```python
from build123d import *

# Parameters (mm, degrees)
SKETCH_1_W          = 1780
SKETCH_1_H          = 100
SKETCH_1_R          = 13
EXTRUDE_573_DEPTH   = 8
SKETCH_2_W          = 1780
SKETCH_2_H          = 8
EXTRUDE_1_DEPTH     = 100
CUT_EXTRUDE_1_DEPTH = 903.088687436


with BuildPart() as part:
    # 草图1 → Extrude 573 (new body)
    with BuildSketch(Plane.XY):
        with Locations((0, 50)):
            Rectangle(SKETCH_1_W, SKETCH_1_H)
        with Locations((840, 40)):
            Circle(SKETCH_1_R, mode=Mode.SUBTRACT)
        with Locations((760, 40)):
            Circle(SKETCH_1_R, mode=Mode.SUBTRACT)
        with Locations(Location((-840, 40, 0), (0, 0, 180))):
            Circle(SKETCH_1_R, mode=Mode.SUBTRACT)
        with Locations(Location((-760, 40, 0), (0, 0, 180))):
            Circle(SKETCH_1_R, mode=Mode.SUBTRACT)
    extrude(amount=EXTRUDE_573_DEPTH)

    # 草图2 → 凸台-拉伸1 (add)
    with BuildSketch(Plane.XY.offset(8)):
        with Locations((0, 96)):
            Rectangle(SKETCH_2_W, SKETCH_2_H)
    extrude(amount=EXTRUDE_1_DEPTH)

    # 草图3 → 切除-拉伸1 (cut, through all)
    with BuildSketch(Plane(origin=(0, 100, 0), x_dir=(-1, 0, 0), z_dir=(0, 1, 0))):
        Polygon((-650, 108), (-890, 0), (-890, 108), align=None)
        Polygon((890, 108), (650, 108), (890, 0), align=None)
    extrude(amount=-CUT_EXTRUDE_1_DEPTH, mode=Mode.SUBTRACT)


solid = part.part
```
Here's how the part is built. I have some questions about the finished solid (model axes, mm). A direction names the side the tool comes from. Coordinates: 2 decimals unless noted, no trailing zeros. Write each loop counter-clockwise with the first axis right and the second up, starting at its lowest first coordinate (ties: lowest second). Pieces come first, ordered by that corner, then holes. Notation, with made-up numbers: (18, -2) - (63, -2) arc R18 cw to (63, 2) - close; hole circle Ø11 at (8, 36). An arc over 180 degrees is marked (long way). One line per item, written item: value.
1) I'm going to push flat-ended pins straight in: P1, Ø3, axis at x = -18.5, z = 67, coming from the -Y side; P2, Ø6, axis at x = 11, y = 59.5, coming from the +Z side. Where does each tip first touch, or does it pass through?
Model answer:
P1: stops at y = 92
P2: stops at z = 8
2) Suppose I cut it at C-C on z = 92. Write out the boundary of the cut face in (x, y), and give its area (3 significant figures).
Model answer:
outline: (-685.56, 92) - (685.56, 92) - (685.56, 100) - (-685.56, 100) - close
area: 11,000 mm²
3) On a 3-axis mill with a long thin cutter (end or side, diameter ignored), from which of +Z, -Z, +X, -X, +Y, -Y can I reach the whole of each face in a straight line? I mean faces 1 (the flat face through (-822.773, 94.678, 30.252)), 2 (the flat face through (-12, 92, 57)). Say none if no direction works.
Model answer:
face 1: +Z, -X, +Y, -Y
face 2: +Z, +X, -X, -Y
4) I need wall thicknesses on line 1 along Y through (x, z) = (760, 3); line 2 along X through (y, z) = (41.5, 5.5); line 3 along Y through (x, z) = (174, 21). Which ranges of each line are inside material? Lowest first, please.
Model answer:
line 1: y = 0 to 27, 53 to 100
line 2: x = -877.78 to -852.91, -827.09 to -772.91, -747.09 to 747.09, 772.91 to 827.09, 852.91 to 877.78
line 3: y = 92 to 100
5) Suppose I cut it at B-B on y = 71.5. Write out the boundary of the cut face in (x, z), and give its area (3 significant figures).
Model answer:
outline: (-890, 0) - (890, 0) - (872.22, 8) - (-872.22, 8) - close
area: 14,100 mm²
6) Suppose I cut it at A-A on x = 51.5. Write out the boundary of the cut face in (y, z), and give its area (3 significant figures).
Model answer:
outline: (0, 0) - (100, 0) - (100, 108) - (92, 108) - (92, 8) - (0, 8) - close
area: 1,600 mm²
